Could you check a few things on this drawing? It's one solid part, dimensions in mm from its lowest x, y, z. A direction names the side the tool comes from. Give positions to 0.01 mm unless a question says otherwise; leave off trailing zeros. Order: outer loops, then holes, each group sorted by start corner. A loop starts at its lowest first (then second) coordinate and runs counter-clockwise, first axis right, second up.
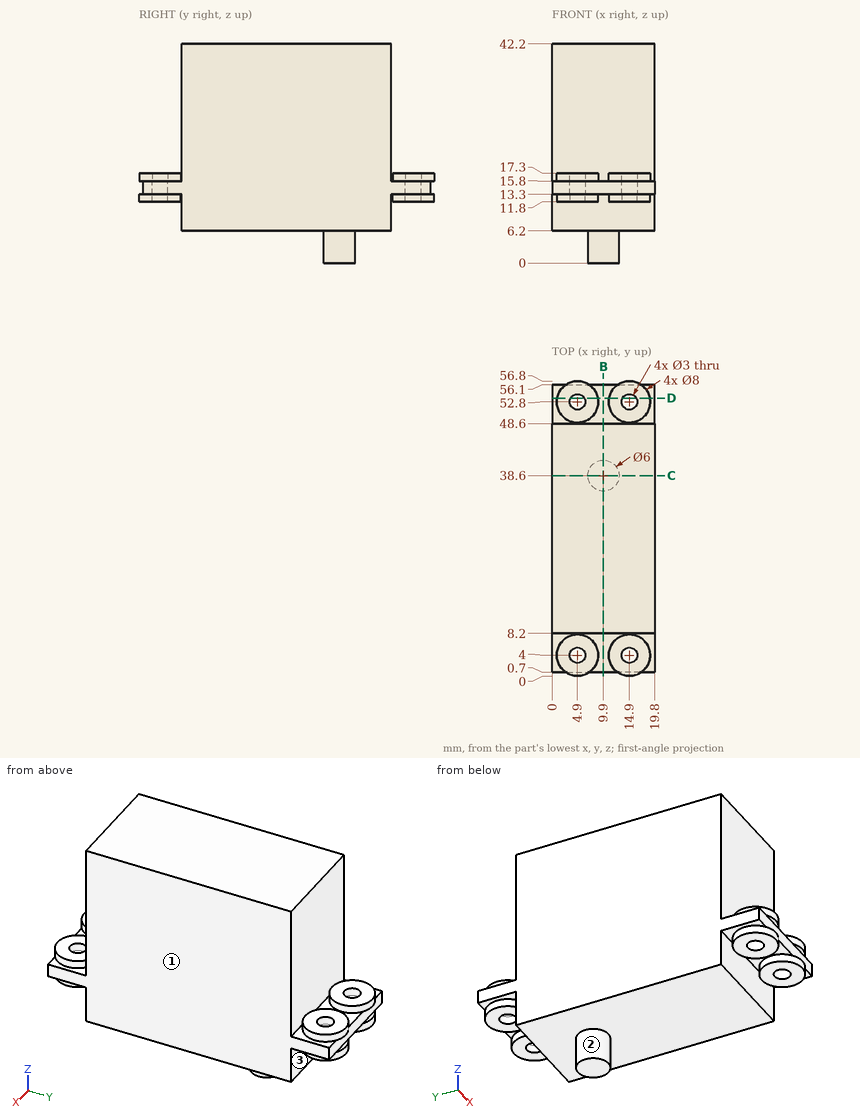
Q1. If we section it at C-C on y = 38.6: List the corners of the cut face in (x, z) for me.
Filled sheet:
outline: (0, 6.2) - (6.9, 6.2) - (6.9, 0) - (12.9, 0) - (12.9, 6.2) - (19.8, 6.2) - (19.8, 42.2) - (0, 42.2) - close
Q2. If we section it at B-B on x = 9.9: List the corners of the cut face in (y, z) for me.
Filled sheet:
outline: (0.7, 13.3) - (8.2, 13.3) - (8.2, 6.2) - (35.6, 6.2) - (35.6, 0) - (41.6, 0) - (41.6, 6.2) - (48.6, 6.2) - (48.6, 13.3) - (56.1, 13.3) - (56.1, 15.8) - (48.6, 15.8) - (48.6, 42.2) - (8.2, 42.2) - (8.2, 15.8) - (0.7, 15.8) - close
Q3. I need wall thicknesses on L1, parallel to Y at x = 14.9, z = 16.9; L2, parallel to X at y = 52.8, z = 15.1; L3, parallel to Z at x = 2, y = 15.5. Which ranges of each line are inside material? Lowest first, please.
Filled sheet:
L1: y = 0 to 2.5, 5.5 to 8, 8.2 to 48.6, 48.8 to 51.3, 54.3 to 56.8
L2: x = 0 to 3.4, 6.4 to 13.4, 16.4 to 19.8
L3: z = 6.2 to 42.2
Q4. I'm going to push flat-ended pins straight in: P1, Ø5.5, axis at x = 12, z = 10.5, coming from the +Y side; P2, Ø4, axis at x = 7.5, y = 52, coming from the -Z side; P3, Ø3.5, axis at x = 14.9, y = 52.8, coming from the +Z side; P4, Ø1.8, axis at x = 4.9, y = 4, coming from the +Z side. Where does each tip first touch, or does it pass through?
Filled sheet:
P1: stops at y = 56.77
P2: stops at z = 11.8
P3: stops at z = 17.3
P4: passes through
Q5. If we section it at D-D on y = 53.5: List the corners of the cut face in (x, z) for me, plus the area to 3 significant figures.
Filled sheet:
outline: (0, 13.3) - (0.96, 13.3) - (0.96, 11.8) - (3.57, 11.8) - (3.57, 17.3) - (0.96, 17.3) - (0.96, 15.8) - (0, 15.8) - close; (6.23, 11.8) - (8.84, 11.8) - (8.84, 13.3) - (10.96, 13.3) - (10.96, 11.8) - (13.57, 11.8) - (13.57, 17.3) - (10.96, 17.3) - (10.96, 15.8) - (8.84, 15.8) - (8.84, 17.3) - (6.23, 17.3) - close; (16.23, 11.8) - (18.84, 11.8) - (18.84, 13.3) - (19.8, 13.3) - (19.8, 15.8) - (18.84, 15.8) - (18.84, 17.3) - (16.23, 17.3) - close
area: 67.6 mm2
Q6. For the marked faces 1, 2 and 3, which set-ups out of +Z, -Z, +X, -X, +Y, -Y let a thin tool reach every point of the face, with its end or its side?
Filled sheet:
face 1: +Z, -Z, +X, +Y, -Y
face 2: -Z
face 3: -Z, +X, -X
